Source: CAD feature listing. Evaluate the final solid. Frame: model axes, mm. Coordinates: 2 decimals unless noted, no trailing zeros. Order: outer loops, then holes, each group sorted by start corner. A loop starts at its lowest first (then second) coordinate and runs counter-clockwise, first axis right, second up.
```python
from build123d import *

# Parameters (mm, degrees)
SKETCH1_R           = 2.4892
SKETCH1_R_2         = 14.2875
SKETCH1_R_3         = 29.9974
BOSS_EXTRUDE1_DEPTH = 3.175
BOSS_EXTRUDE2_START = -3.175
SKETCH2_R           = 2.4892
BOSS_EXTRUDE2_DEPTH = 3.175
FILLET1_R           = 10.16


with BuildPart() as part:
    # Sketch1 → Boss-Extrude1 (new body)
    with BuildSketch(Plane.XY):
        Polygon((-152.4, 0), (152.4, 0), (152.4, 116.084254136), (125.314883545, 190.5), (-152.4, 190.5), align=None)
        with Locations((-139.7, 184.15)):
            Circle(SKETCH1_R, mode=Mode.SUBTRACT)
        with Locations((-127, 184.15)):
            Circle(SKETCH1_R, mode=Mode.SUBTRACT)
        with Locations((-114.3, 184.15)):
            Circle(SKETCH1_R, mode=Mode.SUBTRACT)
        with Locations((-127, 171.45)):
            Circle(SKETCH1_R, mode=Mode.SUBTRACT)
        with Locations((-114.3, 171.45)):
            Circle(SKETCH1_R, mode=Mode.SUBTRACT)
        with Locations((-127, 158.75)):
            Circle(SKETCH1_R, mode=Mode.SUBTRACT)
        with Locations((-114.3, 158.75)):
            Circle(SKETCH1_R, mode=Mode.SUBTRACT)
        with Locations((-127, 146.05)):
            Circle(SKETCH1_R, mode=Mode.SUBTRACT)
        with Locations((-114.3, 146.05)):
            Circle(SKETCH1_R, mode=Mode.SUBTRACT)
        with Locations((-127, 133.35)):
            Circle(SKETCH1_R, mode=Mode.SUBTRACT)
        with Locations((-114.3, 133.35)):
            Circle(SKETCH1_R, mode=Mode.SUBTRACT)
        with Locations((-127, 120.65)):
            Circle(SKETCH1_R, mode=Mode.SUBTRACT)
        with Locations((-114.3, 120.65)):
            Circle(SKETCH1_R, mode=Mode.SUBTRACT)
        with Locations((-127, 107.95)):
            Circle(SKETCH1_R, mode=Mode.SUBTRACT)
        with Locations((-114.3, 107.95)):
            Circle(SKETCH1_R, mode=Mode.SUBTRACT)
        with Locations((-127, 95.25)):
            Circle(SKETCH1_R, mode=Mode.SUBTRACT)
        with Locations((-114.3, 95.25)):
            Circle(SKETCH1_R, mode=Mode.SUBTRACT)
        with Locations((-127, 82.55)):
            Circle(SKETCH1_R, mode=Mode.SUBTRACT)
        with Locations((-114.3, 82.55)):
            Circle(SKETCH1_R, mode=Mode.SUBTRACT)
        with Locations((-127, 69.85)):
            Circle(SKETCH1_R, mode=Mode.SUBTRACT)
        with Locations((-114.3, 69.85)):
            Circle(SKETCH1_R, mode=Mode.SUBTRACT)
        with Locations((-127, 57.15)):
            Circle(SKETCH1_R, mode=Mode.SUBTRACT)
        with Locations((-114.3, 57.15)):
            Circle(SKETCH1_R, mode=Mode.SUBTRACT)
        with Locations((-127, 44.45)):
            Circle(SKETCH1_R, mode=Mode.SUBTRACT)
        with Locations((-114.3, 44.45)):
            Circle(SKETCH1_R, mode=Mode.SUBTRACT)
        with Locations((-127, 31.75)):
            Circle(SKETCH1_R, mode=Mode.SUBTRACT)
        with Locations((-114.3, 31.75)):
            Circle(SKETCH1_R, mode=Mode.SUBTRACT)
        with Locations((-127, 19.05)):
            Circle(SKETCH1_R, mode=Mode.SUBTRACT)
        with Locations((-114.3, 19.05)):
            Circle(SKETCH1_R, mode=Mode.SUBTRACT)
        with Locations((-127, 6.35)):
            Circle(SKETCH1_R, mode=Mode.SUBTRACT)
        with Locations((-114.3, 6.35)):
            Circle(SKETCH1_R, mode=Mode.SUBTRACT)
        with Locations((-139.7, 171.45)):
            Circle(SKETCH1_R, mode=Mode.SUBTRACT)
        with Locations((-139.7, 158.75)):
            Circle(SKETCH1_R, mode=Mode.SUBTRACT)
        with Locations((-139.7, 146.05)):
            Circle(SKETCH1_R, mode=Mode.SUBTRACT)
        with Locations((-139.7, 133.35)):
            Circle(SKETCH1_R, mode=Mode.SUBTRACT)
        with Locations((-139.7, 120.65)):
            Circle(SKETCH1_R, mode=Mode.SUBTRACT)
        with Locations((-139.7, 107.95)):
            Circle(SKETCH1_R, mode=Mode.SUBTRACT)
        with Locations((-139.7, 95.25)):
            Circle(SKETCH1_R, mode=Mode.SUBTRACT)
        with Locations((-139.7, 82.55)):
            Circle(SKETCH1_R, mode=Mode.SUBTRACT)
        with Locations((-139.7, 69.85)):
            Circle(SKETCH1_R, mode=Mode.SUBTRACT)
        with Locations((-139.7, 57.15)):
            Circle(SKETCH1_R, mode=Mode.SUBTRACT)
        with Locations((-139.7, 44.45)):
            Circle(SKETCH1_R, mode=Mode.SUBTRACT)
        with Locations((-139.7, 31.75)):
            Circle(SKETCH1_R, mode=Mode.SUBTRACT)
        with Locations((-139.7, 19.05)):
            Circle(SKETCH1_R, mode=Mode.SUBTRACT)
        with Locations((-139.7, 6.35)):
            Circle(SKETCH1_R, mode=Mode.SUBTRACT)
        with Locations((87.590706137, 182.74937795)):
            Circle(SKETCH1_R, mode=Mode.SUBTRACT)
        with Locations((99.524802421, 187.09303377)):
            Circle(SKETCH1_R, mode=Mode.SUBTRACT)
        with Locations((115.802554525, 179.502593307)):
            Circle(SKETCH1_R, mode=Mode.SUBTRACT)
        with Locations((91.934361957, 170.815281666)):
            Circle(SKETCH1_R, mode=Mode.SUBTRACT)
        with Locations((103.868458241, 175.158937486)):
            Circle(SKETCH1_R, mode=Mode.SUBTRACT)
        with Locations((120.146210345, 167.568497023)):
            Circle(SKETCH1_R, mode=Mode.SUBTRACT)
        with Locations((96.278017777, 158.881185382)):
            Circle(SKETCH1_R, mode=Mode.SUBTRACT)
        with Locations((108.212114061, 163.224841202)):
            Circle(SKETCH1_R, mode=Mode.SUBTRACT)
        with Locations((124.489866165, 155.634400739)):
            Circle(SKETCH1_R, mode=Mode.SUBTRACT)
        with Locations((100.621673597, 146.947089098)):
            Circle(SKETCH1_R, mode=Mode.SUBTRACT)
        with Locations((112.555769881, 151.290744918)):
            Circle(SKETCH1_R, mode=Mode.SUBTRACT)
        with Locations((128.833521986, 143.700304455)):
            Circle(SKETCH1_R, mode=Mode.SUBTRACT)
        with Locations((104.965329418, 135.012992814)):
            Circle(SKETCH1_R, mode=Mode.SUBTRACT)
        with Locations((116.899425702, 139.356648634)):
            Circle(SKETCH1_R, mode=Mode.SUBTRACT)
        with Locations((133.177177806, 131.766208171)):
            Circle(SKETCH1_R, mode=Mode.SUBTRACT)
        with Locations((109.308985238, 123.07889653)):
            Circle(SKETCH1_R, mode=Mode.SUBTRACT)
        with Locations((121.243081522, 127.42255235)):
            Circle(SKETCH1_R, mode=Mode.SUBTRACT)
        with Locations((137.520833626, 119.832111887)):
            Circle(SKETCH1_R, mode=Mode.SUBTRACT)
        with Locations((113.652641058, 111.144800246)):
            Circle(SKETCH1_R, mode=Mode.SUBTRACT)
        with Locations((125.586737342, 115.488456066)):
            Circle(SKETCH1_R, mode=Mode.SUBTRACT)
        with Locations((141.864489446, 107.898015603)):
            Circle(SKETCH1_R, mode=Mode.SUBTRACT)
        with Locations((117.996296878, 99.210703962)):
            Circle(SKETCH1_R, mode=Mode.SUBTRACT)
        with Locations((129.930393162, 103.554359782)):
            Circle(SKETCH1_R, mode=Mode.SUBTRACT)
        with Locations((146.208145266, 95.963919319)):
            Circle(SKETCH1_R, mode=Mode.SUBTRACT)
        with Locations((114.3, 69.85)):
            Circle(SKETCH1_R, mode=Mode.SUBTRACT)
        with Locations((127, 69.85)):
            Circle(SKETCH1_R, mode=Mode.SUBTRACT)
        with Locations((139.7, 69.85)):
            Circle(SKETCH1_R, mode=Mode.SUBTRACT)
        with Locations((114.3, 57.15)):
            Circle(SKETCH1_R, mode=Mode.SUBTRACT)
        with Locations((127, 57.15)):
            Circle(SKETCH1_R, mode=Mode.SUBTRACT)
        with Locations((139.7, 57.15)):
            Circle(SKETCH1_R, mode=Mode.SUBTRACT)
        with Locations((114.3, 44.45)):
            Circle(SKETCH1_R, mode=Mode.SUBTRACT)
        with Locations((127, 44.45)):
            Circle(SKETCH1_R, mode=Mode.SUBTRACT)
        with Locations((139.7, 44.45)):
            Circle(SKETCH1_R, mode=Mode.SUBTRACT)
        with Locations((114.3, 31.75)):
            Circle(SKETCH1_R, mode=Mode.SUBTRACT)
        with Locations((127, 31.75)):
            Circle(SKETCH1_R, mode=Mode.SUBTRACT)
        with Locations((139.7, 31.75)):
            Circle(SKETCH1_R, mode=Mode.SUBTRACT)
        with Locations((114.3, 19.05)):
            Circle(SKETCH1_R, mode=Mode.SUBTRACT)
        with Locations((127, 19.05)):
            Circle(SKETCH1_R, mode=Mode.SUBTRACT)
        with Locations((139.7, 19.05)):
            Circle(SKETCH1_R, mode=Mode.SUBTRACT)
        with Locations((114.3, 6.35)):
            Circle(SKETCH1_R, mode=Mode.SUBTRACT)
        with Locations((127, 6.35)):
            Circle(SKETCH1_R, mode=Mode.SUBTRACT)
        with Locations((139.7, 6.35)):
            Circle(SKETCH1_R, mode=Mode.SUBTRACT)
        with Locations((11.850775283, 132.016841695)):
            Circle(SKETCH1_R_2, mode=Mode.SUBTRACT)
        with Locations((-24.819733341, 71.744857423)):
            Circle(SKETCH1_R_2, mode=Mode.SUBTRACT)
        with Locations((57.635078008, 95.712451111)):
            Circle(SKETCH1_R_2, mode=Mode.SUBTRACT)
        with Locations((23.754601626, 49.678686248)):
            Circle(SKETCH1_R_2, mode=Mode.SUBTRACT)
        with Locations((-65.270180641, 36.953448556)):
            Circle(SKETCH1_R_3, mode=Mode.SUBTRACT)
        with Locations((-65.270180641, 106.549448556)):
            Circle(SKETCH1_R_3, mode=Mode.SUBTRACT)
        with Locations((-7.893480799, 147.995713738)):
            Circle(SKETCH1_R, mode=Mode.SUBTRACT)
        with Locations((31.595031365, 116.037969652)):
            Circle(SKETCH1_R, mode=Mode.SUBTRACT)
        with Locations((5.669801626, 80.209486248)):
            Circle(SKETCH1_R, mode=Mode.SUBTRACT)
        with Locations((41.839401626, 80.209486248)):
            Circle(SKETCH1_R, mode=Mode.SUBTRACT)
        with Locations((41.839401626, 19.147886248)):
            Circle(SKETCH1_R, mode=Mode.SUBTRACT)
        with Locations((5.669801626, 19.147886248)):
            Circle(SKETCH1_R, mode=Mode.SUBTRACT)
    extrude(amount=BOSS_EXTRUDE1_DEPTH)

    # Sketch2 → Boss-Extrude2 (add)
    with BuildSketch(Plane.XY.offset(3.175).offset(BOSS_EXTRUDE2_START)):
        with Locations((146.208145266, 95.963919319)):
            Circle(SKETCH2_R)
    extrude(amount=BOSS_EXTRUDE2_DEPTH)

    # Fillet1
    fillet1_edges = [part.edges().sort_by_distance(p)[0] for p in [
        (-152.4, 190.5, 1.5875),
        (125.314883545, 190.5, 1.5875),
        (152.4, 116.084254136, 1.5875),
        (152.4, 0, 1.5875),
        (-152.4, 0, 1.5875),
    ]]
    fillet(fillet1_edges, radius=FILLET1_R)


solid = part.part
```
1. Section query A-A on x = 68. Return loops of the section in (y, z) (3 decimals), plus the area to 3 significant figures.
Findings:
outline: (0, 0) - (85.879, 0) - (85.879, 3.175) - (0, 3.175) - close; (105.546, 0) - (190.5, 0) - (190.5, 3.175) - (105.546, 3.175) - close
area: 542 mm2
2. Ray query, line 1 (X direction, y = 158.75, z = 1.65); line 2 (X direction, y = 101.5, z = 1); line 3 (Y direction, x = 12, z = 0.7). Return the intervals inside material, ascending.
Findings:
line 1: x = -152.4 to -142.19, -137.21 to -129.49, -124.51 to -116.79, -111.81 to 93.79, 98.76 to 136.87
line 2: x = -152.4 to -94.84, -35.7 to 44.57, 70.7 to 117.02, 118.97 to 128.52, 131.34 to 152.4
line 3: y = 0 to 41.56, 57.8 to 117.73, 146.3 to 190.5
3. Draft query along X for faces 1 (the face through (123.96, 188.71, 1.61)), 2 (the face through (-2, 97, 3.175)), 3 (the face through (18.44, 119.34, 1.57)), 4 (the face through (-149.503, 187.445, 1.61)). Return one class per face: released by +X, released by -X, zero draft, split by the parting line, or undercut.
Findings:
face 1: released by +X
face 2: zero draft
face 3: undercut
face 4: released by -X
4. Section query B-B on z = 0.7. Count the separate pieces of the cut face and the enclosed holes in it, plus the area to 3 significant figures.
Findings:
separate pieces: 1
enclosed holes: 98
area: 47,000 mm2
5. Pin query (flat end, axial travel): P1, Ø4.5, axis at x = 5.67, y = 19.15, coming from the -Z side. Return the tip coordinate at first contact, or that it passes through.
Findings:
P1: passes through
